```python
from build123d import *

# Parameters (mm, degrees)
SKIZZE2_W                            = 26
SKIZZE2_H                            = 26
SCHNITT_LINEAR_AUSTRAGEN1_DEPTH      = 4.7
AUFSATZ_LINEAR_AUSTRAGEN1_DEPTH      = 4.64
AUFSATZ_LINEAR_AUSTRAGEN2_DEPTH      = 1
AUFSATZ_LINEAR_AUSTRAGEN2_DEPTH_BACK = 1


with BuildPart() as part:
    # Skizze1 → Rotation1 (revolve)
    with BuildSketch(Plane.XY, mode=Mode.PRIVATE) as rotation1_sk:
        with BuildLine():
            Line((4.495, 17.9), (4.495, 15.015))
            Line((4.495, 15.015), (6.25, 13.26))
            Line((6.25, 13.26), (6.25, 7.2))
            Line((6.25, 7.2), (5.625, 6.9))
            Line((5.625, 6.9), (6.5, 6.9))
            Line((6.5, 6.9), (7.8, 6.55166605))
            Line((7.8, 6.55166605), (7.8, 2.2))
            Line((7.8, 2.2), (6.5, 2.2))
            Line((6.5, 2.2), (6.5, 1.9))
            Line((6.5, 1.9), (6, 1.9))
            Line((6, 1.9), (6, 1.6))
            Line((6, 1.6), (6.5, 1.6))
            Line((6.5, 1.6), (6.5, 0.3))
            Line((6.5, 0.3), (6, 0.3))
            Line((6, 0.3), (6, 0))
            Line((6, 0), (0, 0))
            Line((0, 0), (0, 22.395))
            ThreePointArc((0, 22.395), (3.178444981, 21.078444981), (4.495, 17.9))
        make_face()
    revolve(rotation1_sk.sketch.rotate(Axis((0, 0, 0), (0, 1, 0)), 270), axis=Axis((0, 0, 0), (0, 1, 0)))

    # Skizze2 → Schnitt-Linear austragen1 (cut)
    with BuildSketch(Plane(origin=(0, 2.2, 0), x_dir=(1, 0, 0), z_dir=(0, 1, 0))):
        Rectangle(SKIZZE2_W, SKIZZE2_H)
        Polygon((-7.505553499, 0), (-3.75277675, -6.5), (3.75277675, -6.5), (7.505553499, 0), (3.75277675, 6.5), (-3.75277675, 6.5), align=None, mode=Mode.SUBTRACT)
    extrude(amount=SCHNITT_LINEAR_AUSTRAGEN1_DEPTH, mode=Mode.SUBTRACT)

    # Skizze3 → Rotation2 (revolve)
    with BuildSketch(Plane.XY, mode=Mode.PRIVATE) as rotation2_sk:
        Polygon((0, 0), (4.864, 0), (4.864, -3.619), (4.283, -4.2), (0, -4.2), align=None)
    revolve(rotation2_sk.sketch.rotate(Axis((0, -4.2, 0), (0, 1, 0)), 270), axis=Axis((0, -4.2, 0), (0, 1, 0)))

    # Skizze4 → Rotation3 (revolve)
    with BuildSketch(Plane(origin=(0, 0, 0), x_dir=(0, 0, -1), z_dir=(1, 0, 0)), mode=Mode.PRIVATE) as rotation3_sk:
        with BuildLine():
            Line((-22.7, 17.9), (-22.7, 22.2))
            Line((-22.7, 22.2), (-22.270691475, 24.634729636))
            ThreePointArc((-22.270691475, 24.634729636), (-22.202287446, 24.753208889), (-22.073729924, 24.8))
            Line((-22.073729924, 24.8), (-21.2, 24.8))
            Line((-21.2, 24.8), (-21.2, 22.95))
            ThreePointArc((-21.2, 22.95), (-21.112132034, 22.737867966), (-20.9, 22.65))
            Line((-20.9, 22.65), (-20.2, 22.65))
            Line((-20.2, 22.65), (-20.2, 24.35))
            Line((-20.2, 24.35), (-19.9, 24.65))
            Line((-19.9, 24.65), (-19.45, 24.65))
            Line((-19.45, 24.65), (-19.35, 24.55))
            Line((-19.35, 24.55), (-19.25, 24.65))
            Line((-19.25, 24.65), (-18.8, 24.65))
            Line((-18.8, 24.65), (-18.7, 24.55))
            Line((-18.7, 24.55), (-18.7, 25.045184441))
            Line((-18.7, 25.045184441), (-16.7, 25.15))
            Line((-16.7, 25.15), (-6.1, 25.15))
            Line((-6.1, 25.15), (-3.345, 22.395))
            Line((-3.345, 22.395), (0, 22.395))
            Line((0, 22.395), (0, 17.9))
            Line((0, 17.9), (-22.7, 17.9))
        make_face()
    revolve(rotation3_sk.sketch.rotate(Axis((0, 17.9, 0), (0, 0, 1)), 270), axis=Axis((0, 17.9, 0), (0, 0, 1)))

    # Skizze5 → Aufsatz-Linear austragen1 (add)
    with BuildSketch(Plane(origin=(0, 17.9, 0), x_dir=(1, 0, 0), z_dir=(0, 1, 0))):
        with BuildLine():
            Line((4.495, -4.34251943), (4.495, 0))
            Line((4.495, 0), (-4.495, 0))
            Line((-4.495, 0), (-4.495, -4.34251943))
            ThreePointArc((-4.495, -4.34251943), (0, -6.25), (4.495, -4.34251943))
        make_face()
    extrude(amount=-AUFSATZ_LINEAR_AUSTRAGEN1_DEPTH)

    # Skizze6 → Aufsatz-Linear austragen2 (add, two sides)
    with BuildSketch(Plane(origin=(0, 0, 0), x_dir=(0, 0, -1), z_dir=(1, 0, 0))) as aufsatz_linear_austragen2_sk:
        Polygon((-11.325, 14.275), (-3.125, 6.075), (-3.125, 14.275), align=None)
    extrude(amount=AUFSATZ_LINEAR_AUSTRAGEN2_DEPTH)
    extrude(aufsatz_linear_austragen2_sk.sketch, amount=-AUFSATZ_LINEAR_AUSTRAGEN2_DEPTH_BACK)

    # Skizze7 → Schnitt-Rotation1 (revolve, cut)
    with BuildSketch(Plane.XY, mode=Mode.PRIVATE) as schnitt_rotation1_sk:
        Polygon((0, 17.9), (3, 17.9), (3, -2.1), (3.242666667, -2.1), (3.242666667, -3.7), (3.742666667, -4.2), (0, -4.2), align=None)
    revolve(schnitt_rotation1_sk.sketch.rotate(Axis((0, -4.2, 0), (0, 1, 0)), 270), axis=Axis((0, -4.2, 0), (0, 1, 0)), mode=Mode.SUBTRACT)

    # Skizze8 → Schnitt-Rotation2 (revolve, cut)
    with BuildSketch(Plane(origin=(0, 0, 0), x_dir=(0, 0, -1), z_dir=(1, 0, 0)), mode=Mode.PRIVATE) as schnitt_rotation2_sk:
        with BuildLine():
            Line((-22.7, 17.9), (-22.7, 22.2))
            ThreePointArc((-22.7, 22.2), (-22.612132034, 21.987867966), (-22.4, 21.9))
            Line((-22.4, 21.9), (-4.6, 21.9))
            Line((-4.6, 21.9), (-4.6, 20.9))
            Line((-4.6, 20.9), (0, 20.9))
            ThreePointArc((0, 20.9), (2.121320344, 20.021320344), (3, 17.9))
            Line((3, 17.9), (-22.7, 17.9))
        make_face()
    revolve(schnitt_rotation2_sk.sketch.rotate(Axis((0, 17.9, 0), (0, 0, 1)), 270), axis=Axis((0, 17.9, 0), (0, 0, 1)), mode=Mode.SUBTRACT)


solid = part.part
```
Input: part model. Units: mm. Frame: model coordinates. A direction names the side the tool comes from. Coordinates: 2 decimals unless noted, no trailing zeros. Write each loop counter-clockwise with the first axis right and the second up, starting at its lowest first coordinate (ties: lowest second). Pieces come first, ordered by that corner, then holes.
1) Set-up query: faces 1 (the flat face through (-4, -4.2, 0)), 2 (the cylindrical face through (0, 8, -3)), 3 (the flat face through (3, 2.2, 6)), 4 (the flat face through (0, 5, -6.5)), 5 (the flat face through (-2, 1.6, -6)). Return all of +Z, -Z, +X, -X, +Y, -Y with unobstructed straight access to the full face (end or side cutting, diameter ignored); none if empty.
2) Mould query, pull axis Z, two halves, no side actions, for faces 6 (the conical face through (-6.744, 6.835, -0.016)), 7 (the cylindrical face through (-0.521, 21.866, 13.375)), 8 (the cylindrical face through (-1.03, 13.263, 20.545)), 9 (the cylindrical face through (-1.46, 11.31, 19.67)). Classes: pulls with the +Z half, pulls with the -Z half, needs draft (parallel to the pull), parting line crosses it, or undercut.
3) Section B-B on y = -1.25. Output: boundary loops of the cut face in (x, z), and give its area (3 significant figures).
4) Material intervals for line 1 along Y through (x, z) = (0.25, 18.5); line 2 along X through (y, z) = (17.9, 1.5) (3 decimals); line 3 along X through (y, z) = (2.5, 0), sorted ascending.
5) Section A-A on z = 14.5. Output: boundary loops of the cut face in (x, y), and give its area (3 significant figures).
6) Pin query (flat end, axial travel): pin 1 Ø1.6 at (x, z) = (-3.5, 4.5) entering from -Y; pin 2 Ø12 at (y, z) = (21, 18) entering from +X; pin 3 Ø10 at (y, z) = (5.5, 10.5) entering from -X. Return the tip coordinate at first contact, or that it passes through.
Check result:
1. face 1: +Z, -Z, +X, -X, -Y
1. face 2: -Y
1. face 3: +Z, +X, -Y
1. face 4: -Z, +X, -X, +Y, -Y
1. face 5: none
2. face 6: parting line crosses it
2. face 7: needs draft
2. face 8: undercut
2. face 9: undercut
3. outline: circle Ø9.73 at (0, 0); hole circle Ø6 at (0, 0)
3. area: 46.1 mm2
4. line 1: y = 10.75 to 13.91, 21.89 to 25.05
4. line 2: x = -4.495 to -3, 3 to 4.495
4. line 3: x = -7.51 to -3, 3 to 7.51
5. outline: circle Ø14.5 at (0, 17.9); hole circle Ø8 at (0, 17.9)
5. area: 115 mm2
6. pin 1: stops at y = 0
6. pin 2: stops at x = 7.25
6. pin 3: stops at x = -4.33
